Part model, mm, in its own coordinate system. A direction names the side the tool comes from. Give positions to 0.01 mm unless a question says otherwise; leave off trailing zeros. Order: outer loops, then holes, each group sorted by start corner. A loop starts at its lowest first (then second) coordinate and runs counter-clockwise, first axis right, second up.
1. Mould opens along X. For faces 3 (the cylindrical face through (13.9, -26.8, 1.6)), 4 (the flat face through (12.6, -14.5, 6.34)), 5 (the cylindrical face through (-15.12, -11.59, 3.21)) say: +X half, -X half, draft (parallel to the pull), parting line (faces both ways), or undercut.
2. Which spindle directions (+Z, -Z, +X, -X, +Y, -Y) get a long thin tool onto all of the face, cutting with end or side? Do faces 1 (the cylindrical face through (23.47, 7.39, 4.74)), 2 (the flat face through (0, -20, 0)). Say none if no direction does.
3. Slice it at A-A on x = 0. List the corners of the cut face in (y, z) (3 decimals).
4. Drop flat-ended pins along their axis: pin 1 Ø3 at (x, z) = (-2.5, 5) entering from +Y; pin 2 Ø2 at (x, y) = (-17.5, 22.5) entering from +Z; pin 3 Ø3 at (x, z) = (3.5, 4.5) entering from +Y. Give the stop position or say it passes through.
5. Slice it at D-D on y = -22. List the corners of the cut face in (x, z), and give its area (3 significant figures).
6. Probe line 1 (Y direction, x = 0, z = 2.25); line 2 (Y direction, x = 0, z = 4) (3 decimals); line 3 (X direction, y = -0.5, z = 1). List the from-to ranges inside material, lowest first.
7. Slice it at C-C on z = 0.75. List the corners of the cut face in (x, y).
from build123d import *

# Parameters (mm, degrees)
SKETCH_R     = 30.19
PAD_DEPTH    = 3.18
SKETCH001_R  = 24.605
PAD001_DEPTH = 6.34
SKETCH002_R  = 19.05
POCKET_DEPTH = 6.341


with BuildPart() as part:
    # Sketch → Pad (new body)
    with BuildSketch(Plane.XY):
        Circle(SKETCH_R)
    extrude(amount=PAD_DEPTH)

    # Sketch001 → Pad001 (join)
    with BuildSketch(Plane.XY):
        Circle(SKETCH001_R)
    extrude(amount=PAD001_DEPTH)

    # Sketch002 (on Face6 of Pad001) → Pocket (cut, through all)
    with BuildSketch(Plane.XY.offset(6.34)):
        Circle(SKETCH002_R)
    extrude(amount=-POCKET_DEPTH, mode=Mode.SUBTRACT)


solid = part.part
Data:
1. face 3: parting line
1. face 4: draft
1. face 5: undercut
2. face 1: +Z
2. face 2: -Z, +X, -X, +Y, -Y
3. outline: (-30.19, 0) - (-19.05, 0) - (-19.05, 6.34) - (-24.605, 6.34) - (-24.605, 3.18) - (-30.19, 3.18) - close; (19.05, 0) - (30.19, 0) - (30.19, 3.18) - (24.605, 3.18) - (24.605, 6.34) - (19.05, 6.34) - close
4. pin 1: stops at y = 24.58
4. pin 2: stops at z = 3.18
4. pin 3: stops at y = 30.06
5. outline: (-20.67, 0) - (20.67, 0) - (20.67, 3.18) - (11.02, 3.18) - (11.02, 6.34) - (-11.02, 6.34) - (-11.02, 3.18) - (-20.67, 3.18) - close
5. area: 201 mm2
6. line 1: y = -30.19 to -19.05, 19.05 to 30.19
6. line 2: y = -24.605 to -19.05, 19.05 to 24.605
6. line 3: x = -30.19 to -19.04, 19.04 to 30.19
7. outline: circle Ø60.38 at (0, 0); hole circle Ø38.1 at (0, 0)
